Verification items for the finished model (mm, model axes). A direction names the side the tool comes from. Give positions to 0.01 mm unless a question says otherwise; leave off trailing zeros. Order: outer loops, then holes, each group sorted by start corner. A loop starts at its lowest first (then second) coordinate and runs counter-clockwise, first axis right, second up. Notation, with made-up numbers: (-2, 33.5) -> (31, 33.5) arc R27 ccw to (31, 56.5) -> close; hole circle Ø9 at (-5, 37.25). An arc over 180 degrees is marked (long way). Return JSON: item names as keys, results as strings. Group by question number.
(1) Cross-section at B-B on y = 31.25. State how many separate pieces and enclosed holes the cut face has, then the cut area to 3 significant figures.
(2) Tool access check on faces 1 (the face through (17.5, 17, 1)), 2 (the face through (6, 5.4, -8)), 3 (the face through (16, 10, 12.5)), 4 (the face through (16, 14.95, 8)). Record the directions out of +Z, -Z, +X, -X, +Y, -Y that give a thin tool (end or side, any length) a straight path to the whole face; none if there is none.
(3) Thickness scan on line 1 along Y through (x, z) = (16.5, 6); line 2 along Z through (x, y) = (9.25, 33.5); line 3 along X through (y, z) = (28.5, 1.75). Record the ranges inside material, lowest first.
(4) Cross-section at A-A on x = 5. Enter the section's corners in (y, z).
(5) Release check for a two-part mould opening along X. For faces 5 (the face through (16.9, 17.74, -8.43)), 6 (the face through (0, 32, -8)), 7 (the face through (13.3, 0, -2.2)), 8 (the face through (3.49, 32.35, -7.99)) record: pulls with the +X half, pulls with the -X half, needs draft (parallel to the pull), parting line crosses it, or undercut.
(6) Cross-section at D-D on z = 15.5. Enter the section's corners in (x, y), then the cut area to 3 significant figures.
(7) Cross-section at C-C on x = 14.5. Enter the section's corners in (y, z).
(8) Depth check by flat-ended pin: pin 1 Ø6 at (y, z) = (33.5, 10.5) entering from -X; pin 2 Ø2 at (y, z) = (18.5, -8.5) entering from -X; pin 3 Ø14 at (y, z) = (16.5, 11.5) entering from +X; pin 4 Ø0.8 at (x, y) = (16.5, 17.5) entering from +Z. Enter the tip coordinate at first touch or a pass-through.
from build123d import *

# Parameters (mm, degrees)
BOSS_EXTRU_1_DEPTH                  = 2.5
ESQUISSE2_W                         = 2.5
ESQUISSE2_H                         = 35
BOSS_EXTRU_2_DEPTH                  = 16
BOSS_EXTRU_3_DEPTH                  = 2
ESQUISSE4_W                         = 2
ESQUISSE4_H                         = 35
BOSS_EXTRU_4_DEPTH                  = 13
ESQUISSE5_W                         = 10
ESQUISSE5_H                         = 5.1
ENL_V_MAT_EXTRU_1_DEPTH             = 2.5
ESQUISSE6_W                         = 11.43
ESQUISSE6_H                         = 24.2
ENL_V_MAT_EXTRU_2_DEPTH             = 3
DIAM_TRE_DU_PER_AGE_2_6_2_6_1_D     = 2.6
DIAM_TRE_DU_PER_AGE_2_6_2_6_1_DEPTH = 28.974295462
DIAM_TRE_DU_PER_AGE_3_0_3_1_D       = 3
DIAM_TRE_DU_PER_AGE_3_0_3_1_DEPTH   = 4.5
CONG_1_R                            = 1
CONG_2_R                            = 2


with BuildPart() as part:
    # Esquisse1 → Boss.-Extru.1 (new body)
    with BuildSketch(Plane(origin=(17.5, 0, 0), x_dir=(0, 0, -1), z_dir=(1, 0, 0))):
        with BuildLine():
            Line((-7, 0), (-7, 35))
            ThreePointArc((-7, 35), (-10.259601203, 33.791437722), (-11.943429983, 30.75))
            ThreePointArc((-11.943429983, 30.75), (-12.14941104, 29.901069836), (-12.5, 29.100946096))
            Line((-12.5, 29.100946096), (-12.5, 5.899053904))
            ThreePointArc((-12.5, 5.899053904), (-12.14941104, 5.098930164), (-11.943429983, 4.25))
            ThreePointArc((-11.943429983, 4.25), (-10.259601203, 1.208562278), (-7, 0))
        make_face()
    extrude(amount=-BOSS_EXTRU_1_DEPTH)

    # Esquisse2 → Boss.-Extru.2 (add)
    with BuildSketch(Plane(origin=(0, 0, 7), x_dir=(-1, 0, 0), z_dir=(0, 0, -1))):
        with Locations((-16.25, 17.5)):
            Rectangle(ESQUISSE2_W, ESQUISSE2_H)
    extrude(amount=BOSS_EXTRU_2_DEPTH)

    # Esquisse3 → Boss.-Extru.3 (add)
    with BuildSketch(Plane.ZY.offset(-15)):
        with BuildLine():
            Line((19.974295462, 21.679625289), (19.974295462, 13.320374711))
            ThreePointArc((19.974295462, 13.320374711), (18.828977674, 10.135814295), (15.917725445, 8.410187356))
            ThreePointArc((15.917725445, 8.410187356), (13.256912127, 6.965462484), (11.917725445, 4.25))
            ThreePointArc((11.917725445, 4.25), (10.233896665, 1.208562278), (6.974295462, 0))
            Line((6.974295462, 0), (-9, 0))
            Line((-9, 0), (-9, 35))
            Line((-9, 35), (6.974295462, 35))
            ThreePointArc((6.974295462, 35), (10.233896665, 33.791437722), (11.917725445, 30.75))
            ThreePointArc((11.917725445, 30.75), (13.256912127, 28.034537516), (15.917725445, 26.589812644))
            ThreePointArc((15.917725445, 26.589812644), (18.828977674, 24.864185705), (19.974295462, 21.679625289))
        make_face()
    extrude(amount=BOSS_EXTRU_3_DEPTH)

    # Esquisse4 → Boss.-Extru.4 (add)
    with BuildSketch(Plane.ZY.offset(-13)):
        with Locations((-8, 17.5)):
            Rectangle(ESQUISSE4_W, ESQUISSE4_H)
    extrude(amount=BOSS_EXTRU_4_DEPTH)

    # Esquisse5 → Enlèv. mat.-Extru.1 (cut)
    with BuildSketch(Plane(origin=(17.5, 0, 0), x_dir=(0, 0, -1), z_dir=(1, 0, 0))):
        with Locations((-7.5, 17.5)):
            Rectangle(ESQUISSE5_W, ESQUISSE5_H)
    extrude(amount=-ENL_V_MAT_EXTRU_1_DEPTH, mode=Mode.SUBTRACT)

    # Esquisse6 → Enlèv. mat.-Extru.2 (cut, through all)
    with BuildSketch(Plane.XY.offset(-7)):
        with Locations((5.715, 17.5)):
            Rectangle(ESQUISSE6_W, ESQUISSE6_H)
    extrude(amount=-ENL_V_MAT_EXTRU_2_DEPTH, mode=Mode.SUBTRACT)

    # Diamètre du perçage Ø2.6 (2.6)1
    with Locations(Plane(origin=(0, 0, -9), x_dir=(-1, 0, 0), z_dir=(0, 0, -1))):
        with Locations((-8.593600322, 3.75), (-8.636, 31.25), (-2.794, 31.25), (-2.836399678, 3.75)):
            Hole(DIAM_TRE_DU_PER_AGE_2_6_2_6_1_D / 2, depth=DIAM_TRE_DU_PER_AGE_2_6_2_6_1_DEPTH)

    # Diamètre du perçage Ø3.0 (3)1
    with Locations(Plane.ZY.offset(-13)):
        with Locations((15.5, 17.5)):
            Hole(DIAM_TRE_DU_PER_AGE_3_0_3_1_D / 2, depth=DIAM_TRE_DU_PER_AGE_3_0_3_1_DEPTH)

    # Congé1
    cong_1_edges = [part.edges().sort_by_distance(p)[0] for p in [
        (13, 17.5, -7),
    ]]
    fillet(cong_1_edges, radius=CONG_1_R)

    # Congé2
    cong_2_edges = [part.edges().sort_by_distance(p)[0] for p in [
        (17.5, 17.5, -9),
    ]]
    fillet(cong_2_edges, radius=CONG_2_R)


solid = part.part
Verdict:
{
 "1": {"separate pieces": "3", "enclosed holes": "0", "area": "109 mm²"},
 "2": {"face 1": "+Z, -Z, +X, +Y, -Y", "face 2": "+Z, -Z, -X", "face 3": "+Z, +X, +Y, -Y", "face 4": "+Z, +X"},
 "3": {"line 1": "0 to 14.95, 20.05 to 35", "line 2": "-9 to -7", "line 3": "13 to 17.5"},
 "4": {"outline": "(0, -9) -> (5.4, -9) -> (5.4, -7) -> (0, -7) -> close; (29.6, -9) -> (35, -9) -> (35, -7) -> (29.6, -7) -> close"},
 "5": {"face 5": "pulls with the +X half", "face 6": "pulls with the -X half", "face 7": "needs draft", "face 8": "undercut"},
 "6": {"outline": "(13, 8.31) -> (15, 8.31) -> (15, 16) -> (13, 16) -> close; (13, 19) -> (15, 19) -> (15, 26.69) -> (13, 26.69) -> close", "area": "30.8 mm²"},
 "7": {"outline": "(0, -9) -> (35, -9) -> (35, 6.97) arc R5 ccw to (30.75, 11.92) arc R5 cw to (26.59, 15.92) arc R5 ccw to (21.68, 19.97) -> (13.32, 19.97) arc R5 ccw to (8.41, 15.92) arc R5 cw to (4.25, 11.92) arc R5 ccw to (0, 6.97) -> close; hole circle Ø3 at (17.5, 15.5)"},
 "8": {"pin 1": "x = 13", "pin 2": "x = 11.43", "pin 3": "x = 17.5", "pin 4": "z = 2.5"}
}
